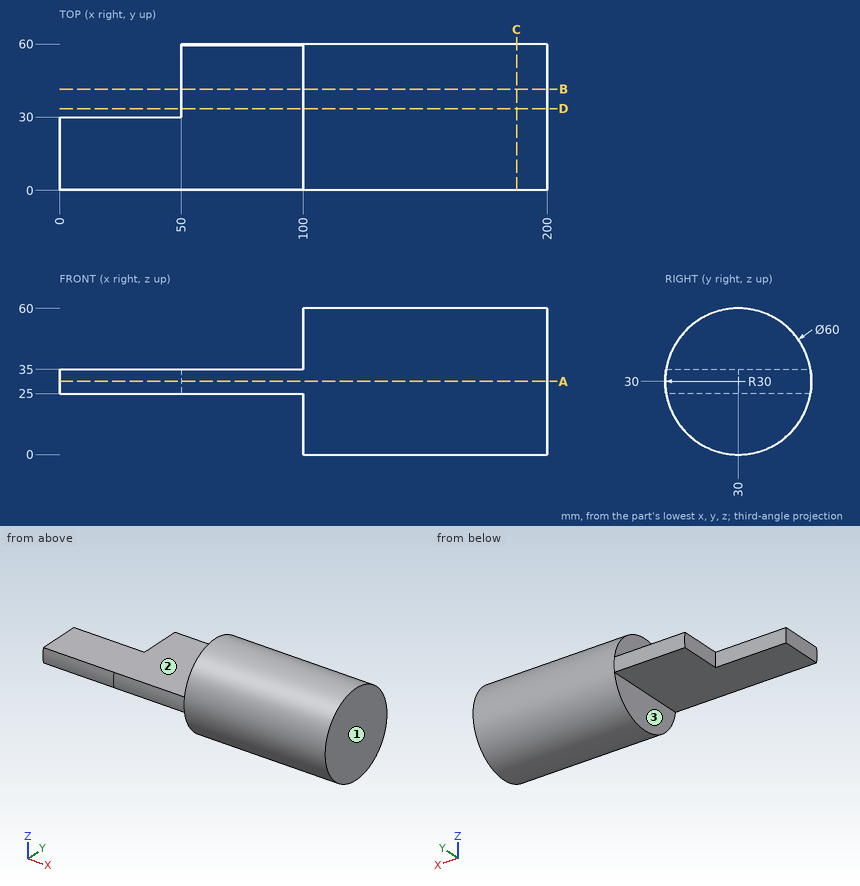
Can you work these out from the drawing? Everything is in mm from the part's minimum corner. A direction names the side the tool comes from. Round coordinates to 2 decimals unless told otherwise and drop trailing zeros. Loops run counter-clockwise (first coordinate to the right, second up) from the corner with the lowest first, then second, coordinate; pieces in that order, holes last. Notation, with made-up numbers: (31, -34.75) - (76, -34.75) arc R23 cw to (76, -14.75) - close; hole circle Ø2 at (-32.5, 31). An arc over 180 degrees is marked (long way). Write item = value, one per line. Start each with the question number.
(1) If I drill on probe 1 along X at (y, z) = (48.5, 43); probe 2 along Z at (x, y) = (75.5, 9); probe 3 along Y at (x, z) = (170, 30), over which ranges is the centre line in solid material (lowest first)? Write a range as [from, to].
(2) For P1, Ø17.5, axis at x = 51, y = 23, coming from the -Z side; P2, Ø2, axis at x = 177.5, z = 31, coming from the +Y side; P3, Ø12.5, axis at y = 43, z = 8.5, coming from the -X side, each with a flat end and sliding along its axis, tell me the tip position at first contact or that it passes through.
(3) If we section it at D-D (y = 33.5): Please give me the cut outline in (x, z).
(4) If we section it at C-C (x = 187.5): Please give me the cut outline in (y, z).
(5) If we section it at A-A (z = 30): Please give me the cut outline in (x, y).
(6) If we section it at B-B (y = 41.5): Please give me the cut outline in (x, z), and give its area (3 significant figures).
(7) For the marked faces 1, 2 and 3, which set-ups out of +Z, -Z, +X, -X, +Y, -Y let a thin tool reach every point of the face, with its end or its side?
Ans:
q1.probe_1 = [100, 200]
q1.probe_2 = [25, 35]
q1.probe_3 = [0, 60]
q2.P1 = 25
q2.P2 = 60
q2.P3 = 100
q3.outline = (50, 25) - (100, 25) - (100, 0.2) - (200, 0.2) - (200, 59.8) - (100, 59.8) - (100, 35) - (50, 35) - close
q4.outline = circle Ø60 at (30, 30)
q5.outline = (0, 0) - (200, 0) - (200, 60) - (50, 60) - (50, 30) - (0, 30) - close
q6.outline = (50, 25) - (100, 25) - (100, 2.29) - (200, 2.29) - (200, 57.71) - (100, 57.71) - (100, 35) - (50, 35) - close
q6.area = 6,040 mm²
q7.face_1 = +Z, -Z, +X, +Y, -Y
q7.face_2 = +Z, -X, +Y, -Y
q7.face_3 = -Z, -X, +Y, -Y
